Check sheet for the modelled part. Datum: model origin and axes. Units: mm. Face numbers are marked on the shaded views. Round coordinates to 2 decimals unless told otherwise and drop trailing zeros. Write each loop counter-clockwise with the first axis right and the second up, starting at its lowest first coordinate (ties: lowest second). Pieces come first, ordered by that corner, then holes. Notation, with made-up numbers: (-8.5, 89.5) -> (30.5, 89.5) arc R25 cw to (30.5, 102.5) -> close; hole circle Ø7 at (60.5, 20). An arc over 180 degrees is marked (long way). One line per item, written item: value.
from build123d import *

# Parameters (mm, degrees)
F1_DEPTH      = 25.4
F2_DEPTH      = 25.4
F3_DEPTH      = 99.822
F3_DEPTH_BACK = 25.4
F4_D          = 6.35
F5_DEPTH      = 127


# Not quite as in the source:
# - a feature names something its author has since deleted; it is built from what else it names


with BuildPart() as f1:
    # F0 (on Front) → F1 (new body)
    with BuildSketch(Plane.XZ):
        with BuildLine():
            Line((32.0781692863, 21.0455041379), (-22.2560535658, 21.0455041379))
            ThreePointArc((-22.2560535658, 21.0455041379), (-26.0561402101, 11.8712834228), (-35.2303609252, 8.0711967784))
            Line((-35.2303609252, 8.0711967784), (-35.2303609252, -36.2501852214))
            Line((-35.2303609252, -36.2501852214), (32.0781692863, -36.2501852214))
            Line((32.0781692863, -36.2501852214), (32.0781692863, 21.0455041379))
        make_face()
        with BuildLine():
            Line((-22.2560535658, 21.0455041379), (-35.2303609252, 21.0455041379))
            Line((-35.2303609252, 21.0455041379), (-35.2303609252, 8.0711967784))
            ThreePointArc((-35.2303609252, 8.0711967784), (-26.0561402101, 11.8712834228), (-22.2560535658, 21.0455041379))
        make_face()
        with BuildLine():
            Line((-35.2303609252, 8.0711967784), (-35.2303609252, 21.0455041379))
            Line((-35.2303609252, 21.0455041379), (-22.2560535658, 21.0455041379))
            ThreePointArc((-22.2560535658, 21.0455041379), (-44.4045816403, 30.2197248529), (-35.2303609252, 8.0711967784))
        make_face()
    extrude(amount=F1_DEPTH)

    # F2 (add): a face of the model
    f2_faces = [f1.faces().sort_by_distance(p)[0] for p in [
        (-4.8856962064, -25.4, -4.7596143665),
    ]]
    extrude(f2_faces, amount=F2_DEPTH)

    # F3 (add, two sides): a face of the model
    f3_faces = [f1.faces().sort_by_distance(p)[0] for p in [
        (4.9110578602, -25.4, 21.0455041379),
    ]]
    extrude(f3_faces, amount=F3_DEPTH)
    extrude(f3_faces, amount=-F3_DEPTH_BACK)

    # F4 (through all)
    with Locations(Plane(origin=(0, 0, 0), x_dir=(1, 0, 0), z_dir=(0, 1, 0))):
        with Locations((-35.2303609252, -21.0455041379)):
            Hole(F4_D / 2)

    # F5 (add): a face of the model
    f5_faces = [f1.faces().sort_by_distance(p)[0] for p in [
        (0.7229147363, 0, 37.7328540078),
    ]]
    extrude(f5_faces, amount=F5_DEPTH)


solid = f1.part
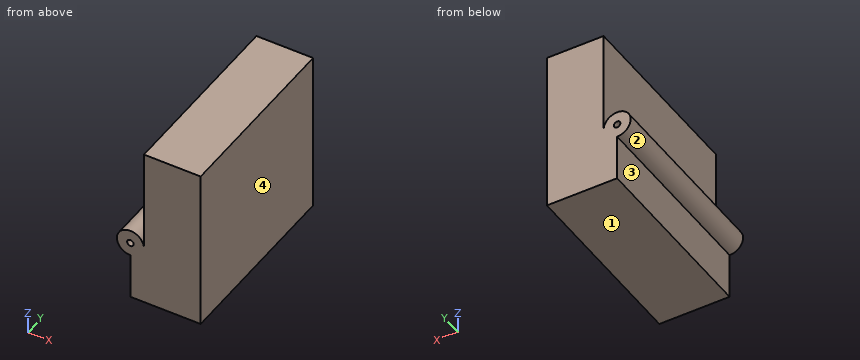
Item 1: Thickness scan on line 1 (X direction, y = 58, z = 99); line 2 (X direction, y = 114.5, z = -8.5); line 3 (X direction, y = -15, z = 19). Record the ranges inside material, lowest first.
Answer:
line 1: x = -22.26 to 32.08
line 2: x = -35.23 to 32.08
line 3: x = -48.04 to -37.66, -32.8 to 32.08
Item 2: Sectioned sample at B-B on z = -7.5. Enter the section's corners in (x, y), and give its area (3 significant figures).
Answer:
outline: (-35.23, -50.8) -> (32.08, -50.8) -> (32.08, 127) -> (-35.23, 127) -> close
area: 12,000 mm^2
Item 3: Mould release check, pull along X, two halves, no side actions. Record for the marked faces 1, 2, 3 and 4: pulls with the +X half, pulls with the -X half, needs draft (parallel to the pull), parting line crosses it, or undercut.
Answer:
face 1: needs draft
face 2: undercut
face 3: pulls with the -X half
face 4: pulls with the +X half
Item 4: Sectioned sample at C-C on z = 105.5. Enter the section's corners in (x, y), and give its area (3 significant figures).
Answer:
outline: (-22.26, -50.8) -> (32.08, -50.8) -> (32.08, 127) -> (-22.26, 127) -> close
area: 9,660 mm^2
Item 5: Depth check by flat-ended pin: P1, Ø4, axis at y = -22.5, z = 18.5, coming from the -X side; P2, Ø3, axis at y = -6, z = -5, coming from the -X side; P3, Ø3, axis at y = 36.5, z = 50, coming from the -X side. Enter the tip coordinate at first touch or a pass-through.
Answer:
P1: stops at x = -48.19
P2: stops at x = -35.23
P3: stops at x = -22.26
